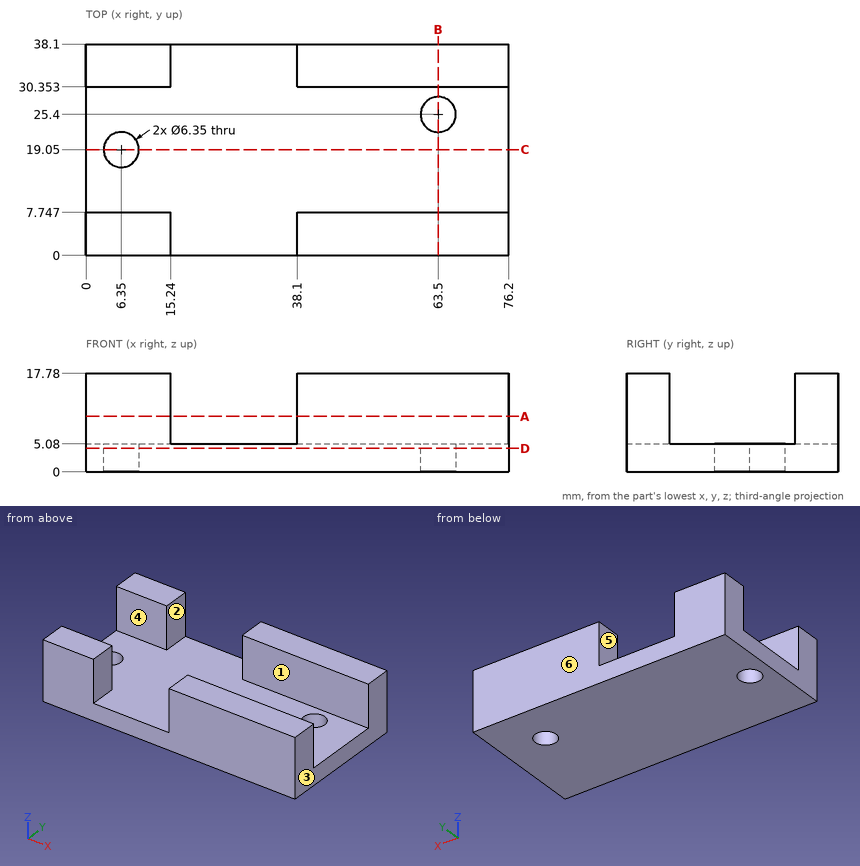
For this review, use the dimensioned drawing (mm, ordinates from the lowest corner) and the shaded views. A direction names the side the tool comes from. Coordinates: 2 decimals unless noted, no trailing zeros. Order: outer loops, then holes, each group sorted by start corner. A loop starts at its lowest first (then second) coordinate and runs counter-clockwise, first axis right, second up. Notation, with made-up numbers: (50, 22.5) - (61, 22.5) arc R16 cw to (61, 44.5) - close; hole circle Ø3 at (-28.75, 57.5). An arc over 180 degrees is marked (long way). Answer as a JSON object with one key per item and string values. Group by question number.
1. For probe 1 along Y at (x, z) = (58, 14.25); probe 2 along Y at (x, z) = (63.5, 2.95) (3 decimals); probe 3 along X at (y, z) = (4.5, 6.5), list the stretches that pass through material, from the lowest coordinate up.
2. We need section C-C on y = 19.05. State the section outline as (x, z) points (3 decimals), then the cut area to 3 significant figures.
3. We need section A-A on z = 10. State the section outline as (x, y) points, then the cut area to 3 significant figures.
4. We need section B-B on x = 63.5. State the section outline as (y, z) points (3 decimals), then the cut area to 3 significant figures.
5. We need section D-D on z = 4.25. State the section outline as (x, y) points (3 decimals), then the cut area to 3 significant figures.
6. For the marked faces 1, 2 and 3, list the 3-axis set-ups (+Z, -Z, +X, -X, +Y, -Y) from which the entire face can be reached by the end or side of a thin tool; tool diameter is ignored.
7. Clearance check with flat-ended pins moving along their axes: P1, Ø4, axis at x = 29.5, y = 12.5, coming from the -Z side; P2, Ø8, axis at x = 68.5, y = 20, coming from the +Z side. State where each tip first meets the part, or that it passes through.
8. The part is to be moulded in two halves that separate along Y. For the marked faces 4, 5 and 6, say which applies: pulls with the +Y half, pulls with the -Y half, needs draft (parallel to the pull), parting line crosses it, or undercut.
Final values:
{
 "1": {"probe 1": "0 to 7.75, 30.35 to 38.1", "probe 2": "0 to 22.225, 28.575 to 38.1", "probe 3": "0 to 15.24, 38.1 to 76.2"},
 "2": {"outline": "(0, 0) - (3.175, 0) - (3.175, 5.08) - (0, 5.08) - close; (9.525, 0) - (76.2, 0) - (76.2, 5.08) - (9.525, 5.08) - close", "area": "355 mm²"},
 "3": {"outline": "(0, 0) - (15.24, 0) - (15.24, 7.75) - (0, 7.75) - close; (0, 30.35) - (15.24, 30.35) - (15.24, 38.1) - (0, 38.1) - close; (38.1, 0) - (76.2, 0) - (76.2, 7.75) - (38.1, 7.75) - close; (38.1, 30.35) - (76.2, 30.35) - (76.2, 38.1) - (38.1, 38.1) - close", "area": "826 mm²"},
 "4": {"outline": "(0, 0) - (22.225, 0) - (22.225, 5.08) - (7.747, 5.08) - (7.747, 17.78) - (0, 17.78) - close; (28.575, 0) - (38.1, 0) - (38.1, 17.78) - (30.353, 17.78) - (30.353, 5.08) - (28.575, 5.08) - close", "area": "358 mm²"},
 "5": {"outline": "(0, 0) - (76.2, 0) - (76.2, 38.1) - (0, 38.1) - close; hole circle Ø6.35 at (6.35, 19.05); hole circle Ø6.35 at (63.5, 25.4)", "area": "2,840 mm²"},
 "6": {"face 1": "+Z, +X, -X", "face 2": "+Z, +Y, -Y", "face 3": "+Z, -Z, +X, +Y, -Y"},
 "7": {"P1": "z = 0", "P2": "z = 5.08"},
 "8": {"face 4": "undercut", "face 5": "needs draft", "face 6": "pulls with the +Y half"}
}
